from build123d import *

# Parameters (mm, degrees)
SKETCH1_R           = 6
BOSS_EXTRUDE1_DEPTH = 2
SKETCH2_R           = 0.75
CUT_EXTRUDE1_DEPTH  = 2
FILLET1_R           = 1.5


with BuildPart() as part:
    # Sketch1 → Boss-Extrude1 (new, symmetric)
    with BuildSketch(Plane.XY):
        Circle(SKETCH1_R)
    extrude(amount=BOSS_EXTRUDE1_DEPTH, both=True)

    # Sketch2 → Cut-Extrude1 (cut, symmetric)
    with BuildSketch(Plane.XY):
        Circle(SKETCH2_R)
    extrude(amount=CUT_EXTRUDE1_DEPTH, both=True, mode=Mode.SUBTRACT)

    # Fillet1
    fillet1_edges = [part.edges().sort_by_distance(p)[0] for p in [
        (-6, 0, -2),
        (-6, 0, 2),
    ]]
    fillet(fillet1_edges, radius=FILLET1_R)


solid = part.part
Design review of the part built by this model. Coordinates are the model's own, in mm. Round coordinates to 2 decimals unless told otherwise and drop trailing zeros. Write each loop counter-clockwise with the first axis right and the second up, starting at its lowest first coordinate (ties: lowest second). Pieces come first, ordered by that corner, then holes.
Item 1: Consider section C-C on z = 0.25. Give the boundary of the cut face in (x, y), and give its area (3 significant figures).
Item 2: For pin 1 Ø1 at (x, y) = (3.5, 4) entering from +Z, flat-tipped, find the tip position at first contact; note if it passes through.
Item 3: Consider section A-A on x = 0. Give the boundary of the cut face in (y, z), and give its area (3 significant figures).
Item 4: Wall thickness on L1, parallel to Y at x = 0, z = 0.2; L2, parallel to Y at x = 0, z = 1; L3, parallel to X at y = -0.5, z = -1.75: over which ranges is each line inside the solid? List them lowest first.
Item 5: Draft analysis for pull direction Y (two halves, no side actions). For faces 1 (the flat face through (0, -1, 2)), 2 (the cylindrical face through (-6, 0, 0)), 3 (the cylindrical face through (-0.75, 0.03, 0.03)), state which applies: released by +Y, released by -Y, zero draft, split by the parting line, or undercut.
Item 6: Consider section D-D on z = 1.2. Give the boundary of the cut face in (x, y).
Check values:
1. outline: circle Ø12 at (0, 0); hole circle Ø1.5 at (0, 0)
1. area: 111 mm2
2. pin 1: stops at z = 1.97
3. outline: (-6, -0.5) arc R1.5 ccw to (-4.5, -2) - (-0.75, -2) - (-0.75, 2) - (-4.5, 2) arc R1.5 ccw to (-6, 0.5) - close; (0.75, -2) - (4.5, -2) arc R1.5 ccw to (6, -0.5) - (6, 0.5) arc R1.5 ccw to (4.5, 2) - (0.75, 2) - close
3. area: 40.1 mm2
4. L1: y = -6 to -0.75, 0.75 to 6
4. L2: y = -5.91 to -0.75, 0.75 to 5.91
4. L3: x = -5.31 to -0.56, 0.56 to 5.31
5. face 1: zero draft
5. face 2: split by the parting line
5. face 3: undercut
6. outline: circle Ø11.65 at (0, 0); hole circle Ø1.5 at (0, 0)
